Geometry check sheet. Reference: the model listing, model coordinates, mm. Give positions to 0.01 mm unless a question says otherwise; leave off trailing zeros. Write each loop counter-clockwise with the first axis right and the second up, starting at its lowest first coordinate (ties: lowest second). Pieces come first, ordered by that corner, then holes. Notation, with made-up numbers: M 8,-6 L 19,-6 A23 ccw 19,6 Z; hole C 81,-38 d6. An arc over 180 degrees is marked long. Use one line per item in the form item = value. Start each with the question number.
```python
from build123d import *

# Parameters (mm, degrees)
PAD001_DEPTH  = 25.4
SKETCH004_R   = 2.1
HOLE001_DEPTH = 195.78938


with BuildPart() as part:
    # CopySketch002 → Pad001 (new body, symmetric)
    with BuildSketch(Plane.XY):
        with BuildLine():
            Line((31.75, 25.4), (-31.75, 25.4))
            Line((-31.75, 25.4), (-31.75, 0))
            Line((-18.225514, 0), (-31.75, 0))
            ThreePointArc((18.225514, 0), (0, 15.325), (-18.225514, 0))
            Line((31.75, 0), (18.225514, 0))
            Line((31.75, 25.4), (31.75, 0))
        make_face()
    extrude(amount=PAD001_DEPTH, both=True)

    # Sketch004 (on Face2 of Pad001) → Hole001 (cut, through all)
    with BuildSketch(Plane(origin=(0, 25.4, 0), x_dir=(-1, 0, 0), z_dir=(0, 1, 0))):
        with Locations((-27.25, 0)):
            Circle(SKETCH004_R)
    hole001 = extrude(amount=-HOLE001_DEPTH, mode=Mode.SUBTRACT)

    # Mirrored002: Hole001 across Sketch004 V_Axis
    add(hole001.mirror(Plane(origin=(0, 25.4, 0), x_dir=(0, 1, 0), z_dir=(-1, 0, 0))), mode=Mode.SUBTRACT)


solid = part.part
```
(1) Thickness scan on probe 1 along Z at (x, y) = (27.25, 15.25); probe 2 along Z at (x, y) = (28.5, 23.25); probe 3 along X at (y, z) = (3.25, 15.5). Record the ranges inside material, lowest first. Write a range as [from, to].
(2) Sectioned sample at A-A, the plane z = 0. Record the boundary of the cut face in (x, y) (3 decimals).
(3) Sectioned sample at D-D, the plane z = 18.5. Record the boundary of the cut face in (x, y) (3 decimals), plus the area to 3 significant figures.
(4) Draft check along X on faces 1 (the flat face through (-24.9, 0, 0.4)), 2 (the flat face through (31.75, 13, 0)), 3 (the cylindrical face through (0.36, 15.32, 0.36)). Enter one of: released by +X, released by -X, zero draft, split by the parting line, or undercut.
(5) Sectioned sample at C-C, the plane x = 27.25. Record the boundary of the cut face in (y, z), plus the area to 3 significant figures.
(6) Depth check by flat-ended pin: pin 1 (6.5 mm diameter, centred on x = -27.25, z = 0, fed in from +Y). Enter the tip coordinate at first touch or a pass-through.
(7) Sectioned sample at B-B, the plane y = 4.25. Record the boundary of the cut face in (x, z), plus the area to 3 significant figures.
Numbers:
q1.probe_1 = [-25.4, -2.1], [2.1, 25.4]
q1.probe_2 = [-25.4, -1.69], [1.69, 25.4]
q1.probe_3 = [-31.75, -17.35], [17.35, 31.75]
q2.outline = M -31.75,0 L -29.35,0 L -29.35,25.4 L -31.75,25.4 Z; M -25.15,0 L -18.226,0 A18.5 cw 18.226,0 L 25.15,0 L 25.15,25.4 L -25.15,25.4 Z; M 29.35,0 L 31.75,0 L 31.75,25.4 L 29.35,25.4 Z
q3.outline = M -31.75,0 L -18.226,0 A18.5 cw 18.226,0 L 31.75,0 L 31.75,25.4 L -31.75,25.4 Z
q3.area = 1,190 mm2
q4.face_1 = zero draft
q4.face_2 = released by +X
q4.face_3 = undercut
q5.outline = M 0,-25.4 L 25.4,-25.4 L 25.4,-2.1 L 0,-2.1 Z; M 0,2.1 L 25.4,2.1 L 25.4,25.4 L 0,25.4 Z
q5.area = 1,180 mm2
q6.pin_1 = 25.4
q7.outline = M -31.75,-25.4 L -16.94,-25.4 L -16.94,25.4 L -31.75,25.4 Z; M 16.94,-25.4 L 31.75,-25.4 L 31.75,25.4 L 16.94,25.4 Z; hole C -27.25,0 d4.2; hole C 27.25,0 d4.2
q7.area = 1,480 mm2
